```python
from build123d import *

# Parameters (mm, degrees)
SKETCH1_W           = 112
SKETCH1_H           = 124
BOSS_EXTRUDE1_DEPTH = 2
SKETCH4_W           = 112
SKETCH4_H           = 124
BOSS_EXTRUDE2_DEPTH = 18
CUT_EXTRUDE1_REACH  = 87.907
SKETCH5_R           = 9.525
SKETCH5_R_2         = 2.5
SKETCH5_W           = 66
SKETCH5_H           = 16
SKETCH6_R           = 2
CUT_EXTRUDE2_DEPTH  = 86.90692638
SKETCH7_R           = 3.5
CUT_EXTRUDE3_DEPTH  = 4
SKETCH8_W           = 50.8
SKETCH8_H           = 20
CUT_EXTRUDE4_DEPTH  = 20


with BuildPart() as part:
    # Sketch1 → Boss-Extrude1 (new body)
    with BuildSketch(Plane(origin=(0, 0, 0), x_dir=(1, 0, 0), z_dir=(0, 1, 0))):
        Rectangle(SKETCH1_W, SKETCH1_H)
    extrude(amount=BOSS_EXTRUDE1_DEPTH)

    # Sketch4 → Boss-Extrude2 (add)
    with BuildSketch(Plane.XZ):
        Rectangle(SKETCH4_W, SKETCH4_H)
        Polygon((-48, 58), (-48, 54), (-52, 54), (-52, -58), (48, -58), (48, -54), (52, -54), (52, 58), align=None, mode=Mode.SUBTRACT)
    extrude(amount=BOSS_EXTRUDE2_DEPTH)

    # Sketch5 → Cut-Extrude1 (cut, up to next)
    with BuildSketch(Plane(origin=(0, 2, 0), x_dir=(1, 0, 0), z_dir=(0, 1, 0)), mode=Mode.PRIVATE) as cut_extrude1_sk1:
        with Locations(Location((-13, 25.1, 0), (0, 0, 270))):
            Circle(SKETCH5_R)
    cut_extrude1_tool1 = extrude(cut_extrude1_sk1.sketch, amount=-CUT_EXTRUDE1_REACH, mode=Mode.PRIVATE) & part.part
    # Sketch5 → Cut-Extrude1 (cut, up to next)
    with BuildSketch(Plane(origin=(0, 2, 0), x_dir=(1, 0, 0), z_dir=(0, 1, 0)), mode=Mode.PRIVATE) as cut_extrude1_sk2:
        with Locations(Location((-46.27, -6.63, 0), (0, 0, 270))):
            Circle(SKETCH5_R_2)
    cut_extrude1_tool2 = extrude(cut_extrude1_sk2.sketch, amount=-CUT_EXTRUDE1_REACH, mode=Mode.PRIVATE) & part.part
    # Sketch5 → Cut-Extrude1 (cut, up to next)
    with BuildSketch(Plane(origin=(0, 2, 0), x_dir=(1, 0, 0), z_dir=(0, 1, 0)), mode=Mode.PRIVATE) as cut_extrude1_sk3:
        with Locations(Location((-34.7, -6.63, 0), (0, 0, 270))):
            Circle(SKETCH5_R_2)
    cut_extrude1_tool3 = extrude(cut_extrude1_sk3.sketch, amount=-CUT_EXTRUDE1_REACH, mode=Mode.PRIVATE) & part.part
    # Sketch5 → Cut-Extrude1 (cut, up to next)
    with BuildSketch(Plane(origin=(0, 2, 0), x_dir=(1, 0, 0), z_dir=(0, 1, 0)), mode=Mode.PRIVATE) as cut_extrude1_sk4:
        with Locations(Location((-21, -12, 0), (0, 0, 270))):
            Circle(SKETCH5_R_2)
    cut_extrude1_tool4 = extrude(cut_extrude1_sk4.sketch, amount=-CUT_EXTRUDE1_REACH, mode=Mode.PRIVATE) & part.part
    # Sketch5 → Cut-Extrude1 (cut, up to next)
    with BuildSketch(Plane(origin=(0, 2, 0), x_dir=(1, 0, 0), z_dir=(0, 1, 0)), mode=Mode.PRIVATE) as cut_extrude1_sk5:
        with Locations(Location((-11, -12, 0), (0, 0, 270))):
            Circle(SKETCH5_R_2)
    cut_extrude1_tool5 = extrude(cut_extrude1_sk5.sketch, amount=-CUT_EXTRUDE1_REACH, mode=Mode.PRIVATE) & part.part
    # Sketch5 → Cut-Extrude1 (cut, up to next)
    with BuildSketch(Plane(origin=(0, 2, 0), x_dir=(1, 0, 0), z_dir=(0, 1, 0)), mode=Mode.PRIVATE) as cut_extrude1_sk6:
        with Locations(Location((9, 30.28, 0), (0, 0, 270))):
            Circle(SKETCH5_R_2)
    cut_extrude1_tool6 = extrude(cut_extrude1_sk6.sketch, amount=-CUT_EXTRUDE1_REACH, mode=Mode.PRIVATE) & part.part
    # Sketch5 → Cut-Extrude1 (cut, up to next)
    with BuildSketch(Plane(origin=(0, 2, 0), x_dir=(1, 0, 0), z_dir=(0, 1, 0)), mode=Mode.PRIVATE) as cut_extrude1_sk7:
        with Locations((2, -37)):
            Rectangle(SKETCH5_W, SKETCH5_H)
    cut_extrude1_tool7 = extrude(cut_extrude1_sk7.sketch, amount=-CUT_EXTRUDE1_REACH, mode=Mode.PRIVATE) & part.part
    add(cut_extrude1_tool1.solids().sort_by_distance((-13, 2, -25.1))[0], mode=Mode.SUBTRACT)
    add(cut_extrude1_tool2.solids().sort_by_distance((-46.27, 2, 6.63))[0], mode=Mode.SUBTRACT)
    add(cut_extrude1_tool3.solids().sort_by_distance((-34.7, 2, 6.63))[0], mode=Mode.SUBTRACT)
    add(cut_extrude1_tool4.solids().sort_by_distance((-21, 2, 12))[0], mode=Mode.SUBTRACT)
    add(cut_extrude1_tool5.solids().sort_by_distance((-11, 2, 12))[0], mode=Mode.SUBTRACT)
    add(cut_extrude1_tool6.solids().sort_by_distance((9, 2, -30.28))[0], mode=Mode.SUBTRACT)
    add(cut_extrude1_tool7.solids().sort_by_distance((2, 2, 37))[0], mode=Mode.SUBTRACT)

    # Sketch6 → Cut-Extrude2 (cut, through all)
    with BuildSketch(Plane(origin=(0, 2, 0), x_dir=(1, 0, 0), z_dir=(0, 1, 0))):
        with Locations(Location((52, 58, 0), (0, 0, 270))):
            Circle(SKETCH6_R)
        with Locations(Location((-52, -58, 0), (0, 0, 270))):
            Circle(SKETCH6_R)
    extrude(amount=-CUT_EXTRUDE2_DEPTH, mode=Mode.SUBTRACT)

    # Sketch7 → Cut-Extrude3 (cut)
    with BuildSketch(Plane(origin=(0, 2, 0), x_dir=(1, 0, 0), z_dir=(0, 1, 0))):
        with Locations(Location((-52, -58, 0), (0, 0, 270))):
            Circle(SKETCH7_R)
        with Locations(Location((52, 58, 0), (0, 0, 270))):
            Circle(SKETCH7_R)
    extrude(amount=-CUT_EXTRUDE3_DEPTH, mode=Mode.SUBTRACT)

    # Sketch8 → Cut-Extrude4 (cut)
    with BuildSketch(Plane.ZY.offset(56)):
        with Locations((-30.25, -8)):
            Rectangle(SKETCH8_W, SKETCH8_H)
    extrude(amount=-CUT_EXTRUDE4_DEPTH, mode=Mode.SUBTRACT)


solid = part.part
```
The model under review builds one solid part; all positions refer to its coordinate system, in mm. A direction names the side the tool comes from. Coordinates: 2 decimals unless noted, no trailing zeros. Write each loop counter-clockwise with the first axis right and the second up, starting at its lowest first coordinate (ties: lowest second). Pieces come first, ordered by that corner, then holes.
1) We need section D-D on x = -46.27. State the section outline as (y, z) points, then the cut area to 3 significant figures.
2) We need section B-B on x = 29. State the section outline as (y, z) points, then the cut area to 3 significant figures.
3) We need section A-A on z = 12. State the section outline as (x, y) points, then the cut area to 3 significant figures.
4) To check wall thickness, follow probe 1 along X at (y, z) = (0.4, 6.63); probe 2 along X at (y, z) = (1.25, 12); probe 3 along Z at (x, y) = (24, -8.75). State the ranges of each line that lie inside material, in increasing order.
5) The part is to be moulded in two halves that separate along X. For faces 4 (the face through (54.365, 0.028, -60.58)), 5 (the face through (-56, -8, 28)), 6 (the face through (-53, -5, -4.85)), 7 (the face through (-37.14, 1.01, 6.09)), say which applies: pulls with the +X half, pulls with the -X half, needs draft (parallel to the pull), parting line crosses it, or undercut.
6) Machinability: for faces 1 (the face through (-49.635, 0.028, 55.42)), 2 (the face through (-50, -9, 54)), 3 (the face through (50, -9, -54)), which of the approach directions +Z, -Z, +X, -X, +Y, -Y give a long, thin tool a straight path to every point of the face, cutting with its end or side? Answer none if there is none.
7) We need section C-C on z = -25.1. State the section outline as (x, y) points (3 decimals).
8) Clearance check with flat-ended pins moving along their axes: pin 1 Ø5 at (x, z) = (33.5, 23.5) entering from -Y; pin 2 Ø4 at (y, z) = (-8, -25) entering from -X; pin 3 Ø3.5 at (x, z) = (51.5, -57.5) entering from +Y; pin 4 Ø4 at (x, z) = (9, -30.28) entering from +Y. State where each tip first meets the part, or that it passes through.
Answer list:
1. outline: (-18, -62) - (2, -62) - (2, -55.65) - (0, -55.65) - (0, -58) - (-18, -58) - close; (-18, 58) - (0, 58) - (0, 9.13) - (2, 9.13) - (2, 62) - (-18, 62) - close; (0, -4.85) - (2, -4.85) - (2, 4.13) - (0, 4.13) - close
1. area: 280 mm2
2. outline: (-18, -62) - (2, -62) - (2, 29) - (0, 29) - (0, -58) - (-18, -58) - close; (-18, 58) - (0, 58) - (0, 45) - (2, 45) - (2, 62) - (-18, 62) - close
2. area: 360 mm2
3. outline: (-56, -18) - (-52, -18) - (-52, 0) - (-23.5, 0) - (-23.5, 2) - (-56, 2) - close; (-18.5, 0) - (-13.5, 0) - (-13.5, 2) - (-18.5, 2) - close; (-8.5, 0) - (52, 0) - (52, -18) - (56, -18) - (56, 2) - (-8.5, 2) - close
3. area: 348 mm2
4. probe 1: x = -56 to -48.77, -43.77 to -37.2, -32.2 to 56
4. probe 2: x = -56 to -23.5, -18.5 to -13.5, -8.5 to 56
4. probe 3: z = -62 to -58, 58 to 62
5. face 4: undercut
5. face 5: pulls with the -X half
5. face 6: needs draft
5. face 7: undercut
6. face 1: +Y
6. face 2: -Y
6. face 3: -X, -Y
7. outline: (-36, 0) - (-22.525, 0) - (-22.525, 2) - (-36, 2) - close; (-3.475, 0) - (52, 0) - (52, -18) - (56, -18) - (56, 2) - (-3.475, 2) - close
8. pin 1: stops at y = 0
8. pin 2: stops at x = 52
8. pin 3: stops at y = -2
8. pin 4: passes through
